Source: CAD feature listing. Evaluate the final solid. Frame: model axes, mm. A direction names the side the tool comes from. Round coordinates to 2 decimals unless told otherwise and drop trailing zeros. Loops run counter-clockwise (first coordinate to the right, second up) from the corner with the lowest first, then second, coordinate; pieces in that order, holes last. Notation, with made-up numbers: (72, 64.25) - (97, 64.25) arc R33 cw to (97, 99.25) - close; hole circle Ø5 at (-37, 45). An arc over 180 degrees is marked (long way). One line per question, with ' | ' between items. Start each with the question number.
1. Cut plane A-A (z = 0). Return loops of the section in (x, y) (1 decimal).
2. Cut plane D-D (x = 11). Return loops of the section in (y, z).
3. Access query for faces 4 (the flat face through (0, 0, 11)), 5 (the flat face through (7.5, -10, -0.2)), 6 (the flat face through (0, 0, -11)), 7 (the flat face through (0, 11, 0)). Directions: +Z, -Z, +X, -X, +Y, -Y. A direction counts if a zero-diameter tool reaches every point of the face in a straight line with its end or side. Return the directions, or none.
4. Ray query, line 1 (X direction, y = -1.5, z = 3); line 2 (X direction, y = 0.25, z = 5.75); line 3 (Y direction, x = 17.5, z = -9.5). Return the intervals inside material, ascending.
5. Cut plane B-B (y = 0). Return loops of the section in (x, z) (1 decimal).
6. Cut plane C-C (x = -16.5). Return loops of the section in (y, z), then the cut area to 3 significant figures.
7. Pin query (flat end, axial travel): pin 1 (1 mm diameter, centred on x = 17.5, y = 4.5, fed in from +Z); pin 2 (1.5 mm diameter, centred on y = -0.5, z = -7, fed in from +X); pin 3 (7 mm diameter, centred on x = -20, y = -4.5, fed in from +Z); pin 4 (1.5 mm diameter, centred on x = 18.5, z = -6, fed in from -Y). Return the tip coordinate at first contact, or that it passes through.
8. Mould query, pull axis Y, two halves, no side actions, for faces 1 (the flat face through (-8, 11.906, 0)), 2 (the cylindrical face through (27.78, 0.14, 0.26)), 3 (the cylindrical face through (-23.805, 0.349, -0.14)). Classes: pulls with the +Y half, pulls with the -Y half, needs draft (parallel to the pull), parting line crosses it, or undercut.
```python
from build123d import *

# Parameters (mm, degrees)
SKETCH3_R           = 7.9375
BOSS_EXTRUDE2_DEPTH = 10
SKETCH4_R           = 11.90625
SKETCH4_R_2         = 7.9375
BOSS_EXTRUDE3_DEPTH = 10


with BuildPart() as part:
    # Sketch3 → Boss-Extrude2 (new, symmetric)
    with BuildSketch(Plane.XY):
        with BuildLine():
            Line((0, -11.90625), (0, 11.90625))
            Line((0, 11.90625), (-15.875, 11.90625))
            ThreePointArc((-15.875, 11.90625), (-27.78125, 0), (-15.875, -11.90625))
            Line((-15.875, -11.90625), (0, -11.90625))
        make_face()
        with Locations((-15.875, 0)):
            Circle(SKETCH3_R, mode=Mode.SUBTRACT)
    extrude(amount=BOSS_EXTRUDE2_DEPTH, both=True)

    # Sketch4 → Boss-Extrude3 (add, symmetric)
    with BuildSketch(Plane(origin=(0, 0, 0), x_dir=(1, 0, 0), z_dir=(0, 1, 0))):
        with Locations((15.875, 0)):
            Circle(SKETCH4_R)
        with Locations(Location((15.875, 0, 0), (0, 0, 270))):
            Circle(SKETCH4_R_2, mode=Mode.SUBTRACT)
        with BuildLine():
            Line((0, -11.90625), (15.875, -11.90625))
            ThreePointArc((15.875, -11.90625), (3.96875, 0), (15.875, 11.90625))
            Line((15.875, 11.90625), (0, 11.90625))
            Line((0, 11.90625), (0, -11.90625))
        make_face()
    extrude(amount=BOSS_EXTRUDE3_DEPTH, both=True)


solid = part.part
```
Answers follow:
1) outline: (-15.9, -11.9) - (0, -11.9) - (0, -10) - (7.9, -10) - (7.9, 10) - (0, 10) - (0, 11.9) - (-15.9, 11.9) arc R11.9 ccw to start; (23.8, -10) - (27.8, -10) - (27.8, 10) - (23.8, 10) - close; hole circle Ø15.9 at (-15.9, 0)
2) outline: (-10, -11.91) - (10, -11.91) - (10, -6.26) - (-10, -6.26) - close; (-10, 6.26) - (10, 6.26) - (10, 11.91) - (-10, 11.91) - close
3) face 4: +Z, -X, +Y, -Y | face 5: +Z, -Z, +X, -Y | face 6: -Z, -X, +Y, -Y | face 7: +Z, -Z, +X, +Y
4) line 1: x = -27.69 to -23.67, -8.08 to 8.53, 23.22 to 27.4 | line 2: x = -27.78 to -23.81, -7.94 to 10.4, 21.35 to 26.3 | line 3: y = -10 to 10
5) outline: (-27.8, -10) - (-23.8, -10) - (-23.8, 10) - (-27.8, 10) - close; (-7.9, -10) - (0, -10) - (0, -11.9) - (15.9, -11.9) arc R11.9 ccw to (15.9, 11.9) - (0, 11.9) - (0, 10) - (-7.9, 10) - close; hole circle Ø15.9 at (15.9, 0)
6) outline: (-11.89, -10) - (-7.91, -10) - (-7.91, 10) - (-11.89, 10) - close; (7.91, -10) - (11.89, -10) - (11.89, 10) - (7.91, 10) - close | area: 159 mm2
7) pin 1: stops at z = 11.85 | pin 2: stops at x = 26.01 | pin 3: stops at z = 10 | pin 4: passes through
8) face 1: pulls with the +Y half | face 2: needs draft | face 3: undercut
